Can you work these out from the model? Positions are in its coordinate system, mm. Face numbers are marked on the shaded views. A direction names the side the tool comes from. Coordinates: 2 decimals unless noted, no trailing zeros. Order: outer loops, then holes, each group sorted by start corner. A loop starts at its lowest first (then second) coordinate and runs counter-clockwise, first axis right, second up. Notation, with made-up numbers: (34.5, 45) -> (46.5, 45) arc R10 ccw to (46.5, 53) -> close; hole circle Ø9 at (85, 5). An arc over 180 degrees is marked (long way). Answer in a Markdown table with one row per item. Add a question column.
1. Imagine slicing it at A-A on z = -2.75. Write out the boundary of the cut face in (x, y), plus the area to 3 significant figures.
2. On a 3-axis mill with a long thin cutter (end or side, diameter ignored), from which of +Z, -Z, +X, -X, +Y, -Y can I reach the whole of each face in a straight line? I mean the marked faces 5, 6 and 7. Say none if no direction works.
3. Imagine slicing it at C-C on x = -17.5. Write out the boundary of the cut face in (y, z), plus the area to 3 significant figures.
4. Imagine slicing it at D-D on z = -26.8. Write out the boundary of the cut face in (x, y).
5. We'd pull the mould along X, two halves only. Please class the marked faces 1, 2, 3 and 4: pulls with the +X half, pulls with the -X half, needs draft (parallel to the pull), parting line crosses it, or undercut.
6. If I drill on line 1 along Z through (x, y) = (-4.75, 0.5); line 2 along X through (y, z) = (0.4, -37.25); line 3 along X through (y, z) = (0.4, -2.75), over which ranges is the centre line in solid material (lowest first)? Write a range as [from, to].
7. Will these pins go through, and if not, where does the flat tip stop? pin 1 (3 mm diameter, centred on x = -4, y = 7, fed in from -Z); pin 2 (3 mm diameter, centred on y = 5, z = -15, fed in from +X); pin 3 (7.5 mm diameter, centred on x = 11.5, z = -11, fed in from +Y).
8. Imagine slicing it at B-B on x = -4.75. Write out the boundary of the cut face in (y, z), plus the area to 3 significant figures.
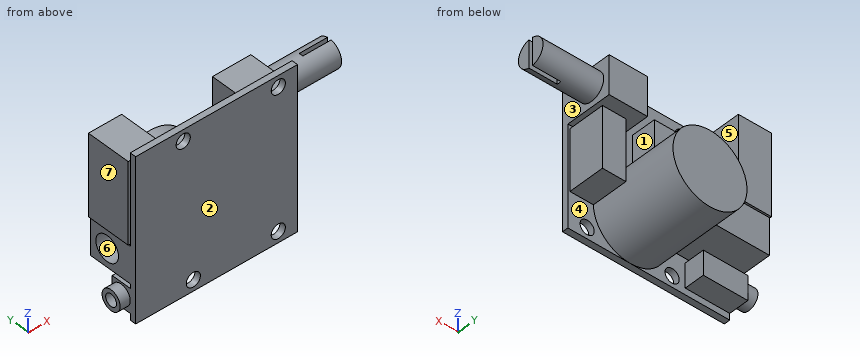
Autodesk Inventor part; units mm, degrees
ref_plane "YZ Plane" through (0, 0, 0) normal (1, 0, 0) x (0, 1, 0)
ref_plane "XZ Plane" through (0, 0, 0) normal (0, 1, 0) x (-1, 0, 0)
ref_plane "XY Plane" through (0, 0, 0) normal (0, 0, 1) x (1, 0, 0)
sketch "Sketch1" plane through (0, 0, 0) normal (0, 1, 0) x (-1, 0, 0)
  line L0 (0, 0) -> (40, 0)
  line L1 (40, 0) -> (40, -40)
  line L2 (40, -40) -> (0, -40)
  line L3 (0, -40) -> (0, 0)
  dimension "d0" = 40
  dimension "d1" = 40
extrude "Extrusion1" add sketch "Sketch1" along normal blind 1.5
sketch "Sketch2" plane through (0, 1.5, 0) normal (0, 1, 0) x (1, 0, 0)
  circle A0 centre (-4.75, 37.25) radius 1.75
  circle A1 centre (-25.75, 37.25) radius 1.75
  circle A2 centre (-28.25, 2.75) radius 1.75
  circle A3 centre (-4.75, 2.75) radius 1.75
  circle A4 centre (-15.45, 30.85) radius 9.15
  line L0 (-40, 32.4) -> (-29, 32.4)
  line L1 (-29, 32.4) -> (-29, 38.4)
  line L2 (-29, 38.4) -> (-40, 38.4)
  line L3 (-40, 38.4) -> (-40, 32.4)
  line L4 (-40.5, 31.3) -> (-26.5, 31.3)
  line L5 (-26.5, 31.3) -> (-26.5, 22.3)
  line L6 (-26.5, 22.3) -> (-40.5, 22.3)
  line L7 (-40.5, 22.3) -> (-40.5, 31.3)
  line L8 (-40.5, 21.8) -> (-32.3, 21.8)
  line L9 (-32.3, 21.8) -> (-32.3, 1.8)
  line L10 (-32.3, 1.8) -> (-40.5, 1.8)
  line L11 (-40.5, 1.8) -> (-40.5, 21.8)
  line L12 (-9.5, 15.15) -> (0, 15.15)
  line L13 (0, 15.15) -> (0, 5.6)
  line L14 (0, 5.6) -> (-9.5, 5.6)
  line L15 (-9.5, 5.6) -> (-9.5, 15.15)
  line L16 (-6.3, 31) -> (-0.5, 31)
  line L17 (-0.5, 31) -> (-0.5, 16)
  line L18 (-0.5, 16) -> (-6.3, 16)
  line L19 (-6.3, 16) -> (-6.3, 31)
  line L20 (-25.2, 17.8) -> (-16, 17.8)
  line L21 (-16, 17.8) -> (-16, 9)
  line L22 (-16, 9) -> (-25.2, 9)
  line L23 (-25.2, 9) -> (-25.2, 17.8)
  line L24 (-40, 0) -> (0, 0)
  line L25 (0, 40) -> (-40, 40)
  line L26 (-40, 40) -> (-40, 0)
  line L27 (-40, 0) -> (0, 0)
  line L28 (0, 0) -> (0, 40)
  line L29 (0, 40) -> (-40, 40)
  point P0 (-36.4, 1.8)
  point P1 (-40, 31.3)
  point P2 (-40, 22.3)
  dimension "d4" = 3.5
  dimension "d5" = 3.5
  dimension "d6" = 3.5
  dimension "d7" = 3.5
  dimension "d8" = 18.3
  dimension "d9" = 8.2
  dimension "d10" = 20
  dimension "d11" = 8.8
  dimension "d12" = 9.2
  dimension "d13" = 9.55
  dimension "d14" = 9.5
  dimension "d15" = 15
  dimension "d16" = 5.8
  dimension "d17" = 11
  dimension "d18" = 6
  dimension "d21" = 9
  dimension "d22" = 14
  dimension "d23" = 5.6
  dimension "d24" = 4.75
  dimension "d25" = 2.75
  dimension "d26" = 0.5
  dimension "d27" = 9
  dimension "d28" = 9
  dimension "d29" = 6.5
  dimension "d30" = 9.15
  dimension "d31" = 9.15
  dimension "d32" = 2.75
  dimension "d33" = 0.5
  dimension "d34" = 1.8
  dimension "d35" = 1.6
  dimension "d37" = 0.5
  dimension "d38" = 0.5
  dimension "d39" = 11.75
  dimension "d40" = 2.75
  dimension "d41" = 2.75
  dimension "d42" = 4.75
  dimension "d43" = 14.25
extrude "Extrusion2" add sketch "Sketch2" along normal blind 6 contours L20 L21 L22 L23
extrude "Extrusion3" add sketch "Sketch2" along normal blind 22 contours A4
extrude "Extrusion4" cut sketch "Sketch2" against normal through all contours A0 | A1 | A2 | A3
extrude "Extrusion5" add sketch "Sketch2" along normal blind 11 contours L26 L8 L9 L10 | L10 L11 L8 L26
extrude "Extrusion6" add sketch "Sketch2" along normal blind 11.4 contours L13 L14 L15 L12
sketch "Sketch2 outline for Extrusion7" plane through (0, 1.5, 0) normal (0, 1, 0) x (1, 0, 0)
  line L0 (-6.3, 16) -> (-0.5, 16)
  line L1 (-6.3, 31) -> (-6.3, 16)
  line L2 (-0.5, 31) -> (-6.3, 31)
  line L3 (-0.5, 16) -> (-0.5, 31)
extrude "Extrusion7" add sketch "Sketch2 outline for Extrusion7" along normal blind 9
extrude "Extrusion8" add sketch "Sketch2" along normal blind 11 contours L4 L5 L6 L26
extrude "Extrusion9" add sketch "Sketch2" along normal blind 5 contours L2 L1 L0 L3
sketch "Sketch3" plane through (-40, 0, -40) normal (-1, 0, 0) x (0, 0, 1)
  line L0 (8.7, 12.5) -> (17.7, 12.5)
  line L1 (8.7, 1.5) -> (8.7, 12.5)
  line L2 (17.7, 1.5) -> (17.7, 12.5)
  circle A0 centre (13.2, 7.875) radius 3.125
  point P0 (40, 0)
  dimension "d60" = 6.25
  dimension "d61" = 4.625
extrude "Extrusion10" cut sketch "Sketch3" against normal blind 13
sketch "Sketch4" plane through (-40, 0, -40) normal (-1, 0, 0) x (0, 0, 1)
  line L0 (1.6, 1.5) -> (1.6, 6.5)
  line L1 (1.6, 6.5) -> (7.6, 6.5)
  line L2 (7.6, 1.5) -> (7.6, 6.5)
  circle A0 centre (4.6, 4) radius 2.5
  circle A1 centre (4.6, 4) radius 1.5
  point P0 (40, 0)
  dimension "d64" = 5
  dimension "d65" = 1
  dimension "d66" = 6
  dimension "d67" = 3
extrude "Extrusion11" add sketch "Sketch4" along normal blind 2.5
sketch "Sketch5" plane through (0, 0, 0) normal (1, 0, 0) x (0, 0, -1)
  circle A0 centre (10.375, 8) radius 3.4
  line L0 (15.15, 1.5) -> (15.15, 12.9)
  line L1 (5.6, 12.9) -> (15.15, 12.9)
  line L2 (5.6, 1.5) -> (5.6, 12.9)
  point P0 (0, 0)
  dimension "d70" = 6.8
  dimension "d71" = 4.9
  dimension "d72" = 4.775
  dimension "d73" = 9.55
extrude "Extrusion12" add sketch "Sketch5" along normal blind 15
sketch "Sketch6" plane through (15, 8, -10.375) normal (1, 0, 0) x (0, 0, -1)
  circle A0 centre (0, 0) radius 3.4
  line L0 (-3.363034, 0.5) -> (3.363034, 0.5)
  line L1 (3.363034, 0.5) -> (3.363034, -0.5)
  line L2 (3.363034, -0.5) -> (-3.363034, -0.5)
  line L3 (-3.363034, -0.5) -> (-3.363034, 0.5)
  line L4 (-3.363034, 0.5) -> (3.363034, -0.5) construction
  line L5 (3.363034, 0.5) -> (-3.363034, -0.5) construction
  point P0 (-3.363034, 0.5)
  point P1 (-3.363034, -0.5)
  point P2 (3.363034, 0.5)
  dimension "d76" = 1
extrude "Extrusion13" cut sketch "Sketch6" against normal blind 7 contours A0 L1 | L1 L2 L3 L0 | L3 A0
equation "\"d5\" = d4"
equation "\"d6\" = d5"
equation "\"d7\" = d4"
equation "\"d30\" = 0.5 * d8"
equation "\"d31\" = 0.5 * d8"
properties part number "amp"
Answers follow:
| question | item | result |
|---|---|---|
| 1 | outline | (-40.5, 1.5) -> (-40, 1.5) -> (-40, 0) -> (-30, 0) -> (-30, 1.5) -> (-32.3, 1.5) -> (-32.3, 12.5) -> (-40.5, 12.5) -> close; (-26.5, 0) -> (-6.5, 0) -> (-6.5, 1.5) -> (-26.5, 1.5) -> close; (-3, 0) -> (0, 0) -> (0, 1.5) -> (-3, 1.5) -> close |
| 1 | area | 140 mm² |
| 2 | face 5 | +Z, +Y |
| 2 | face 6 | -X |
| 2 | face 7 | +Z, -X, +Y, -Y |
| 3 | outline | (0, -40) -> (1.5, -40) -> (1.5, -39.77) -> (23.5, -39.77) -> (23.5, -21.93) -> (1.5, -21.93) -> (1.5, -17.8) -> (7.5, -17.8) -> (7.5, -9) -> (1.5, -9) -> (1.5, 0) -> (0, 0) -> close |
| 3 | area | 505 mm² |
| 4 | outline | (-40, 0) -> (0, 0) -> (0, 1.5) -> (-0.5, 1.5) -> (-0.5, 10.5) -> (-6.3, 10.5) -> (-6.3, 1.5) -> (-7.25, 1.5) -> (-7.25, 23.5) -> (-23.65, 23.5) -> (-23.65, 1.5) -> (-26.5, 1.5) -> (-26.5, 12.5) -> (-40, 12.5) -> (-40, 11) -> (-27, 11) -> (-27, 4.75) -> (-40, 4.75) -> close |
| 5 | face 1 | undercut |
| 5 | face 2 | needs draft |
| 5 | face 3 | pulls with the +X half |
| 5 | face 4 | undercut |
| 6 | line 1 | z = [-40, -39], [-35.5, -4.5], [-1, 0] |
| 6 | line 2 | x = [-40, -27.5], [-24, -6.5], [-3, 0] |
| 6 | line 3 | x = [-40, -30], [-26.5, -6.5], [-3, 0] |
| 7 | pin 1 | stops at z = -31 |
| 7 | pin 2 | stops at x = 0 |
| 7 | pin 3 | stops at y = 11.4 |
| 8 | outline | (0, -40) -> (1.5, -40) -> (1.5, -39) -> (0, -39) -> close; (0, -35.5) -> (1.5, -35.5) -> (1.5, -31) -> (10.5, -31) -> (10.5, -16) -> (1.5, -16) -> (1.5, -15.15) -> (12.9, -15.15) -> (12.9, -5.6) -> (1.5, -5.6) -> (1.5, -4.5) -> (0, -4.5) -> close; (0, -1) -> (1.5, -1) -> (1.5, 0) -> (0, 0) -> close |
| 8 | area | 293 mm² |
